Autodesk Fusion 360 part; units mm, degrees
sketch "Sketch1" plane through (0, 0, 0) normal (1, 0, 0) x (0, 1, 0)
  circle A0 centre (0, 0) radius 1.225
  circle A1 centre (0, 0) radius 2.25
  line L0 (0, -2.25) -> (-7, -2.25)
  line L1 (-7, -2.25) -> (-7, -0.25)
  line L2 (-7, -0.25) -> (0, -0.25)
  line L3 (0, -0.25) -> (0, -2.25)
  line L4 (-4.9672, 4.6123) -> (6.1553, 4.6123)
  line L5 (6.1553, 4.6123) -> (6.1553, 0.8852)
  line L6 (6.1553, 0.8852) -> (-4.9672, 0.8852)
  line L7 (-4.9672, 0.8852) -> (-4.9672, 4.6123)
  line L8 (0, -2.25) -> (2.25, -2.25)
  line L9 (2.25, -2.25) -> (2.25, 0)
  line L10 (2.25, 0) -> (0, 0)
  line L11 (0, 0) -> (0, -2.25)
  dimension "d1" = 2.45
  dimension "d2" = 4.5
  dimension "d3" = 7
  dimension "d4" = 2
  dimension "d5" = 2.25
  dimension "d6" = 2.25
extrude "Extrude1" add sketch "Sketch1" along normal blind 8 contours A0 A1 L3 L10 L11 | A0 A1 L6 L10 | A0 A1 L2 L3 L11 | A1 L8 L9 | A0 A1 L2 L6 | A1 L0 L1 L2
sketch "Sketch2" plane through (0, 0, 0) normal (0, 0, 1) x (1, 0, 0)
  circle A0 centre (4, -4.5) radius 1.25
  dimension "d9" = 2.5
extrude "Extrude2" cut sketch "Sketch2" against normal blind 6.5
chamfer "Chamfer1" distance 1 angle 45 1 edges at (2.8346, -4.048, -0.25)
fillet "Fillet1" radius 2 2 edges at (0, -7, -1.25) (8, -7, -1.25)
The model under review builds one solid part; all positions refer to its coordinate system, in mm. Round coordinates to 2 decimals unless told otherwise and drop trailing zeros. Order: outer loops, then holes, each group sorted by start corner. A loop starts at its lowest first (then second) coordinate and runs counter-clockwise, first axis right, second up. Notation, with made-up numbers: (40.5, 4.25) - (58.5, 4.25) arc R26 ccw to (58.5, 19.25) - close; hole circle Ø7 at (1.5, 44.25). An arc over 180 degrees is marked (long way). Use one line per item in the form item = value.
Q1. Add section A-A on y = -4.5. Give the boundary of the cut face in (x, z).
Response values:
outline = (0, -2.25) - (2.75, -2.25) - (2.75, -1.25) - (1.75, -0.25) - (0, -0.25) - close; (5.25, -2.25) - (8, -2.25) - (8, -0.25) - (6.25, -0.25) - (5.25, -1.25) - close
Q2. Add section D-D on x = 1. Give the boundary of the cut face in (y, z) (3 decimals).
Response values:
outline = (-6.732, -2.25) - (2.25, -2.25) - (2.25, 0) arc R2.25 ccw to (2.069, 0.885) - (0.847, 0.885) arc R1.225 cw (long way) to (-0.847, 0.885) - (-2.069, 0.885) arc R2.25 ccw to (-2.236, -0.25) - (-6.732, -0.25) - close
Q3. Add section C-C on z = 0.7. Give the boundary of the cut face in (x, y), then the cut area to 3 significant figures.
Response values:
outline = (0, -2.14) - (8, -2.14) - (8, -1.01) - (0, -1.01) - close; (0, 1.01) - (8, 1.01) - (8, 2.14) - (0, 2.14) - close
area = 18.1 mm^2
Q4. Clearance check with flat-ended pins moving along their axes: P1, Ø2, axis at x = 5, y = -3.5, coming from the +Z side; P2, Ø1.5, axis at x = 4, y = -4.5, coming from the +Z side. State where each tip first meets the part, or that it passes through.
Response values:
P1 = -0.25
P2 = through
Q5. To check wall thickness, follow line 1 (Y direction, x = 2.5, z = 0) (3 decimals); line 2 (Y direction, x = 4, z = -1.9); line 3 (Y direction, x = 3, z = -0.8). State the ranges of each line that lie inside material, in increasing order.
Response values:
line_1 = -2.25 to -1.225, 1.225 to 2.25
line_2 = -7 to -5.75, -3.25 to 2.25
line_3 = -7 to -5.87, -3.13 to -0.93, 0.93 to 2.25
Q6. Add section B-B on z = -1.9. Give the boundary of the cut face in (x, y).
Response values:
outline = (0, -5) arc R2 ccw to (2, -7) - (6, -7) arc R2 ccw to (8, -5) - (8, 2.25) - (0, 2.25) - close; hole circle Ø2.5 at (4, -4.5)
Q7. Mouldability with a two-part tool opening along Y and no side actions: class faces 1 (the flat face through (4, 2.25, -1)), 2 (the flat face through (4, -2, -2.25)), 3 (the cylindrical face through (3.944, 0.041, -1.224)) as pulls with the +Y half, pulls with the -Y half, needs draft (parallel to the pull), parting line crosses it, or undercut.
Response values:
face_1 = pulls with the +Y half
face_2 = needs draft
face_3 = undercut
